from build123d import *

# Parameters (mm, degrees)
EXTRUDE_DEPTH = 79


with BuildPart() as obj1:
    # Part__Mirroring → Extrude (new body)
    with BuildSketch(Plane(origin=(-25, -1.004737, 0), x_dir=(0, 1, 0), z_dir=(0, 0, 1))):
        with BuildLine():
            ThreePointArc((14.004737, -25), (11.372036, -17.156587), (4.540257, -12.49))
            Line((4.540257, -12.49), (-4.000791, -5))
            Line((-4.000791, -5), (-4.004737, 25))
            Line((-4.004737, 25), (-14.004737, 25))
            Line((-14.004737, 25), (-14.004737, -25))
            Line((-14.004737, -25), (-2.745263, -25))
            ThreePointArc((-2.745263, -25), (1.004737, -21.25), (4.754737, -25))
            Line((4.754737, -25), (14.004737, -25))
        make_face()
    extrude(amount=EXTRUDE_DEPTH)


with BuildPart() as fusion:
    # Part__Mirroring001: instance of obj1
    add(obj1.part.mirror(Plane(origin=(0, 0, 0), x_dir=(0, -1, 0), z_dir=(1, 0, 0))))

    # Fusion: union obj1
    add(obj1.part)


solid = fusion.part
The listing builds one solid part. Answer for the finished solid, in the listing's coordinates (mm). Give positions to 0.01 mm unless a question says otherwise; leave off trailing zeros. Loops run counter-clockwise (first coordinate to the right, second up) from the corner with the lowest first, then second, coordinate; pieces in that order, holes last. Notation, with made-up numbers: (-40, 36.25) - (-35, 36.25) arc R14 ccw to (-35, 43.25) - close; hole circle Ø7 at (85.5, -11.5). An arc over 180 degrees is marked (long way). Answer as a JSON object with one key per item and string values.
1. A cutting plane is placed at C-C (x = 25). Write down the section's boundary in (y, z), then the cut area to 3 significant figures.
Determined:
{"outline": "(-15.01, 0) - (-5.01, 0) - (-5.01, 79) - (-15.01, 79) - close", "area": "790 mm²"}
2. A cutting plane is placed at B-B (y = -2.5). Write down the section's boundary in (x, z), then the cut area to 3 significant figures.
Determined:
{"outline": "(-17.8, 0) - (-2.8, 0) - (-2.8, 79) - (-17.8, 79) - close; (2.8, 0) - (17.8, 0) - (17.8, 79) - (2.8, 79) - close", "area": "2,370 mm²"}
3. A cutting plane is placed at D-D (y = 9.5). Write down the section's boundary in (x, z), then the cut area to 3 significant figures.
Determined:
{"outline": "(-8.87, 0) - (8.87, 0) - (8.87, 79) - (-8.87, 79) - close", "area": "1,400 mm²"}
4. Find the intervals of material crossed by L1, parallel to Y at x = 0, z = 23.5; L2, parallel to X at y = 0, z = 30; L3, parallel to X at y = -2.5, z = 20.5, in increasing order. Write a range as [from, to].
Determined:
{"L1": "[-15.01, -3.75], [3.75, 13]", "L2": "[-15.61, -3.75], [3.75, 15.61]", "L3": "[-17.8, -2.8], [2.8, 17.8]"}
5. For a pull along X with two mould halves and no side action, classify faces 1 (the flat face through (50, -10, 39)), 2 (the cylindrical face through (-3.66, 0.81, 38.95)), 3 (the flat face through (-1, -7, 0)) as pulls with the +X half, pulls with the -X half, needs draft (parallel to the pull), parting line crosses it, or undercut.
Determined:
{"face 1": "pulls with the +X half", "face 2": "undercut", "face 3": "needs draft"}
6. A cutting plane is placed at A-A (z = 47.5). Write down the section's boundary in (x, y), then the cut area to 3 significant figures.
Determined:
{"outline": "(-50, -15.01) - (50, -15.01) - (50, -5.01) - (20, -5.01) - (12.51, 3.54) arc R13 ccw to (0, 13) arc R13 ccw to (-12.51, 3.54) - (-20, -5.01) - (-50, -5.01) - close; hole circle Ø7.5 at (0, 0)", "area": "1,410 mm²"}
7. Flat-ended cylindrical pins translate along their axes: pin 1 Ø15 at (x, z) = (39, 25.5) entering from +Y; pin 2 Ø1 at (y, z) = (9, 11) entering from -X; pin 3 Ø4 at (y, z) = (4, 20.5) entering from +X; pin 4 Ø3 at (x, y) = (18.5, 1) entering from -Z. Find the tip coordinate at first contact, or state that the pin passes through.
Determined:
{"pin 1": "y = -5.01", "pin 2": "x = -9.84", "pin 3": "x = 13.86", "pin 4": "through"}
